```python
from build123d import *

# Parameters (mm, degrees)
F1_DEPTH = 20
F2_R     = 2.75
F3_DEPTH = 25
F2_R_2   = 5
F4_DEPTH = 28.4
F5_DEPTH = 5
F2_W     = 20
F2_H     = 5.6
F6_DEPTH = 3


with BuildPart() as f1:
    # F0 (on Top) → F1 (new body)
    with BuildSketch(Plane.XY):
        Polygon((-3.25, 17.5), (-10, 17.5), (-10, -17.5), (10, -17.5), (10, 17.5), (3.25, 17.5), (3.25, 15.8), (5.15, 15.8), (5.15, 14.3), (3.25, 11), (-3.25, 11), (-5.15, 14.3), (-5.15, 15.8), (-3.25, 15.8), align=None)
        Polygon((10, 17.5), (10, -17.5), (30, -17.5), align=None)
    extrude(amount=F1_DEPTH)

    # F2 (on face) → F3 (cut)
    with BuildSketch(Plane.XZ.offset(17.5)):
        with Locations((20, 10)):
            Circle(F2_R)
    extrude(amount=-F3_DEPTH, mode=Mode.SUBTRACT)

    # F2 (on face) → F4 (cut)
    with BuildSketch(Plane.XZ.offset(17.5)):
        with Locations((20, 10)):
            Circle(F2_R_2)
        with Locations((20, 10)):
            Circle(F2_R, mode=Mode.SUBTRACT)
    extrude(amount=-F4_DEPTH, mode=Mode.SUBTRACT)

    # F2 (on face) → F5 (join)
    with BuildSketch(Plane.XZ.offset(17.5)):
        with Locations((20, 10)):
            Circle(F2_R_2)
        with Locations((20, 10)):
            Circle(F2_R, mode=Mode.SUBTRACT)
    extrude(amount=-F5_DEPTH)

    # F2 (on face) → F6 (join)
    with BuildSketch(Plane.XZ.offset(17.5)):
        with Locations((0, 10)):
            Rectangle(F2_W, F2_H)
    extrude(amount=F6_DEPTH)


solid = f1.part
```
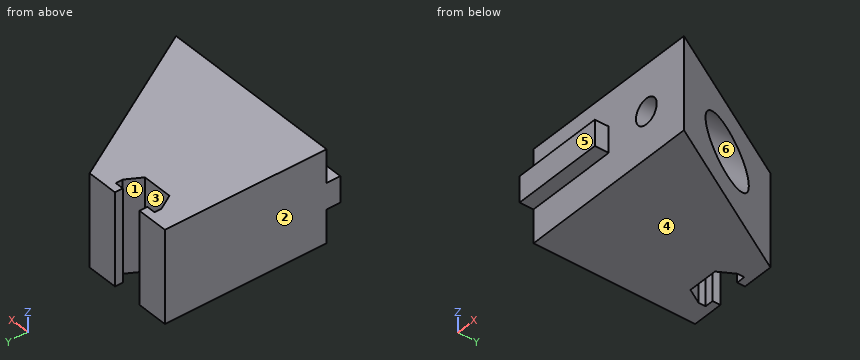
The model under review builds one solid part; all positions refer to its coordinate system, in mm. Face numbers are marked on the shaded views. A direction names the side the tool comes from. Coordinates: 2 decimals unless noted, no trailing zeros. Write each loop counter-clockwise with the first axis right and the second up, starting at its lowest first coordinate (ties: lowest second). Pieces come first, ordered by that corner, then holes.
1) To check wall thickness, follow probe 1 along Z at (x, y) = (20, -13.5); probe 2 along Z at (x, y) = (20, -4); probe 3 along Y at (x, z) = (20, 1). State the ranges of each line that lie inside material, in increasing order.
2) The part is to be moulded in two halves that separate along Z. For the marked faces 4, 5 and 6, say which applies: pulls with the +Z half, pulls with the -Z half, needs draft (parallel to the pull), parting line crosses it, or undercut.
3) Clearance check with flat-ended pins moving along their axes: pin 1 Ø7 at (x, z) = (-0.5, 11.5) entering from +Y; pin 2 Ø3.5 at (x, y) = (-3, -19.5) entering from -Z; pin 3 Ø12 at (y, z) = (-8, 9.5) entering from +X; pin 4 Ø5 at (x, z) = (17, 4.5) entering from -Y. State where each tip first meets the part, or that it passes through.
4) We need section C-C on z = 4.5. State the section outline as (x, y) points.
5) We need section A-A on z = 10. State the section outline as (x, y) points.
6) Machinability: for the marked faces 1, 2 and 3, which of the approach directions +Z, -Z, +X, -X, +Y, -Y give a long, thin tool a straight path to every point of the face, cutting with its end or side? Answer none if there is none.
7) We need section D-D on y = -9.5. State the section outline as (x, z) points.
8) We need section B-B on x = 20. State the section outline as (y, z) points.
Answer list:
1. probe 1: z = 0 to 7.25, 12.75 to 20
1. probe 2: z = 0 to 5, 15 to 20
1. probe 3: y = -17.5 to 0
2. face 4: pulls with the -Z half
2. face 5: needs draft
2. face 6: undercut
3. pin 1: stops at y = 17.5
3. pin 2: stops at z = 7.2
3. pin 3: stops at x = 28
3. pin 4: stops at y = -17.5
4. outline: (-10, -17.5) - (30, -17.5) - (10, 17.5) - (3.25, 17.5) - (3.25, 15.8) - (5.15, 15.8) - (5.15, 14.3) - (3.25, 11) - (-3.25, 11) - (-5.15, 14.3) - (-5.15, 15.8) - (-3.25, 15.8) - (-3.25, 17.5) - (-10, 17.5) - close
5. outline: (-10, -20.5) - (10, -20.5) - (10, -17.5) - (17.25, -17.5) - (17.25, -12.5) - (15, -12.5) - (15, 8.75) - (10, 17.5) - (3.25, 17.5) - (3.25, 15.8) - (5.15, 15.8) - (5.15, 14.3) - (3.25, 11) - (-3.25, 11) - (-5.15, 14.3) - (-5.15, 15.8) - (-3.25, 15.8) - (-3.25, 17.5) - (-10, 17.5) - close; (22.75, -17.5) - (30, -17.5) - (25, -8.75) - (25, -12.5) - (22.75, -12.5) - close
6. face 1: +Z, -Z
6. face 2: +Z, -Z, -X, +Y, -Y
6. face 3: +Z, -Z, +Y
7. outline: (-10, 0) - (25.43, 0) - (25.43, 20) - (-10, 20) - close; hole circle Ø10 at (20, 10)
8. outline: (-17.5, 0) - (0, 0) - (0, 5) - (-12.5, 5) - (-12.5, 7.25) - (-17.5, 7.25) - close; (-17.5, 12.75) - (-12.5, 12.75) - (-12.5, 15) - (0, 15) - (0, 20) - (-17.5, 20) - close
